Part model, mm, in its own coordinate system. Face numbers are marked on the shaded views. Round coordinates to 2 decimals unless told otherwise and drop trailing zeros. Order: outer loops, then holes, each group sorted by start corner. A loop starts at its lowest first (then second) coordinate and runs counter-clockwise, first axis right, second up. Notation, with made-up numbers: (52.5, 80.5) - (91.5, 80.5) arc R27 cw to (91.5, 102.5) - close; hole circle Ø7 at (-27, 16.25). An arc over 180 degrees is marked (long way). Answer as a JSON object with one key per item and string values.
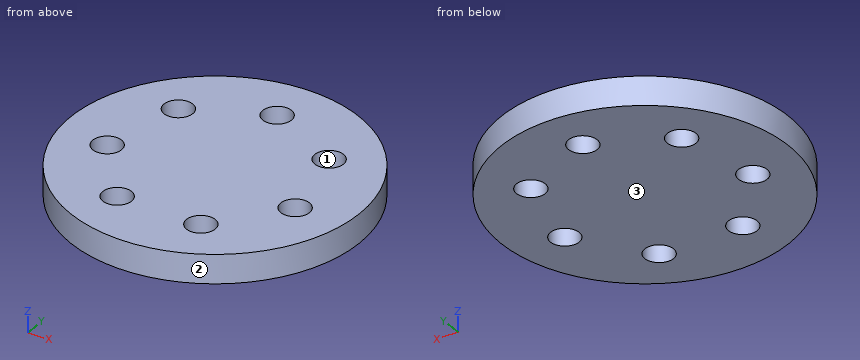
```python
from build123d import *

# Parameters (mm, degrees)
F2_R            = 65
F3_DEPTH        = 13
F4_R            = 6.5
F5_DEPTH        = 13.001
F5_COPIES_COUNT = 7


# Not quite as in the source:
# - a pattern or mirror of a feature is missing from the dataset's text; its kind, count and spacing are read off the source's solid


with BuildPart() as f3:
    # F2 (on Top) → F3 (new body)
    with BuildSketch(Plane.XY):
        Circle(F2_R)
    extrude(amount=F3_DEPTH)

    # F4 (on face) → F5 (cut, through all)
    with BuildSketch(Plane.XY.offset(13)):
        with Locations((0, 43.3333333333)):
            Circle(F4_R)
    f5 = extrude(amount=-F5_DEPTH, mode=Mode.SUBTRACT)

    # F5_copies: F5 ×7 about axis
    f5_copies_axis = Axis((0, 0, 0), (0, 0, 1))
    for i in range(1, F5_COPIES_COUNT):
        add(f5.rotate(f5_copies_axis, i * 360 / F5_COPIES_COUNT), mode=Mode.SUBTRACT)


solid = f3.part
```
Item 1: Two-plate mould, pull along Y, no slides. Class the marked faces 1, 2 and 3: pulls with the +Y half, pulls with the -Y half, needs draft (parallel to the pull), parting line crosses it, or undercut.
Taken from the geometry:
{"face 1": "undercut", "face 2": "parting line crosses it", "face 3": "needs draft"}
Item 2: Drop flat-ended pins along their axis: P1, Ø1.5, axis at x = 38.5, z = 3.5, coming from the -Y side; P2, Ø5, axis at x = -50.5, z = 6.5, coming from the +Y side; P3, Ø8, axis at x = 33.88, y = 27.02, coming from the -Z side; P4, Ø2, axis at y = 13, z = 9, coming from the +X side. Give the stop position or say it passes through.
Taken from the geometry:
{"P1": "y = -52.91", "P2": "y = 43.83", "P3": "through", "P4": "x = 63.88"}
Item 3: Cut at A-A (y = 24.5). Write the cut outline in (x, z).
Taken from the geometry:
{"outline": "(-60.21, 0) - (-39.87, 0) - (-39.87, 13) - (-60.21, 13) - close; (-27.89, 0) - (27.89, 0) - (27.89, 13) - (-27.89, 13) - close; (39.87, 0) - (60.21, 0) - (60.21, 13) - (39.87, 13) - close"}
Item 4: Cut at C-C (z = 8.75). Write the cut outline in (x, y), plus the area to 3 significant figures.
Taken from the geometry:
{"outline": "circle Ø130 at (0, 0); hole circle Ø13 at (-42.25, -9.64); hole circle Ø13 at (-33.88, 27.02); hole circle Ø13 at (-18.8, -39.04); hole circle Ø13 at (0, 43.33); hole circle Ø13 at (18.8, -39.04); hole circle Ø13 at (33.88, 27.02); hole circle Ø13 at (42.25, -9.64)", "area": "12,300 mm2"}
Item 5: Cut at B-B (x = 0). Write the cut outline in (y, z).
Taken from the geometry:
{"outline": "(-65, 0) - (36.83, 0) - (36.83, 13) - (-65, 13) - close; (49.83, 0) - (65, 0) - (65, 13) - (49.83, 13) - close"}
Item 6: Probe L1, parallel to X at y = -15, z = 4.75; L2, parallel to X at y = -41, z = 8.25; L3, parallel to Y at x = 38, z = 5.5. List the from-to ranges inside material, lowest first. Write a range as from..to.
Taken from the geometry:
{"L1": "-63.25..-45.93, -38.57..38.57, 45.93..63.25", "L2": "-50.44..-25, -12.6..12.6, 25..50.44", "L3": "-52.74..-14.56, -4.72..21.99, 32.04..52.74"}
Item 7: Cut at D-D (x = 45.5). Write the cut outline in (y, z).
Taken from the geometry:
{"outline": "(-46.42, 0) - (-15.27, 0) - (-15.27, 13) - (-46.42, 13) - close; (-4.02, 0) - (46.42, 0) - (46.42, 13) - (-4.02, 13) - close"}
